Job drawing, mm, ordinate dimensions from the low corner. One solid piece. A direction names the side the tool comes from. Give positions to 0.01 mm unless a question says otherwise; leave off trailing zeros. Order: outer loops, then holes, each group sorted by start corner. A loop starts at its lowest first (then second) coordinate and runs counter-clockwise, first axis right, second up. Notation, with made-up numbers: (-2, -30) - (16, -30) arc R13 cw to (16, -12) - close; hole circle Ø8 at (-4.75, 57.25). An arc over 180 degrees is marked (long way). Use one line per item in the form item = value. Start each with the question number.
1. Band-saw the part on C-C, the plane z = 14.75. List the corners of the cut face in (x, y).
2. Band-saw the part on B-B, the plane x = 23. List the corners of the cut face in (y, z), plus the area to 3 significant figures.
3. Band-saw the part on A-A, the plane y = 23. List the corners of the cut face in (x, z), plus the area to 3 significant figures.
4. Pin check, flat tips, straight feed: P1, Ø1, axis at x = 7, z = 3, coming from the +Y side; P2, Ø2, axis at x = 23.5, z = 17, coming from the +Y side; P3, Ø6, axis at y = 22, z = 3.5, coming from the -X side. Stop position of each tip, or through.
5. Band-saw the part on D-D, the plane z = 6. List the corners of the cut face in (x, y).
6. Pull direction Y, two halves, no side cores. Call the marked faces 4, 5, 6 and 7: +Y half, -Y half, draft (parallel to the pull), parting line (faces both ways), or undercut.
7. Tool access for the marked faces 1, 2 and 3: list every direction of +Z, -Z, +X, -X, +Y, -Y with a clear straight run to the whole face (end or side of a thin tool).
8. Drill centre lines: line 1 (X direction, y = 27, z = 6.25); line 2 (Y direction, x = 23, z = 18.5); line 3 (Y direction, x = 23, z = 12.65). Where is each one in solid material? Low to high.
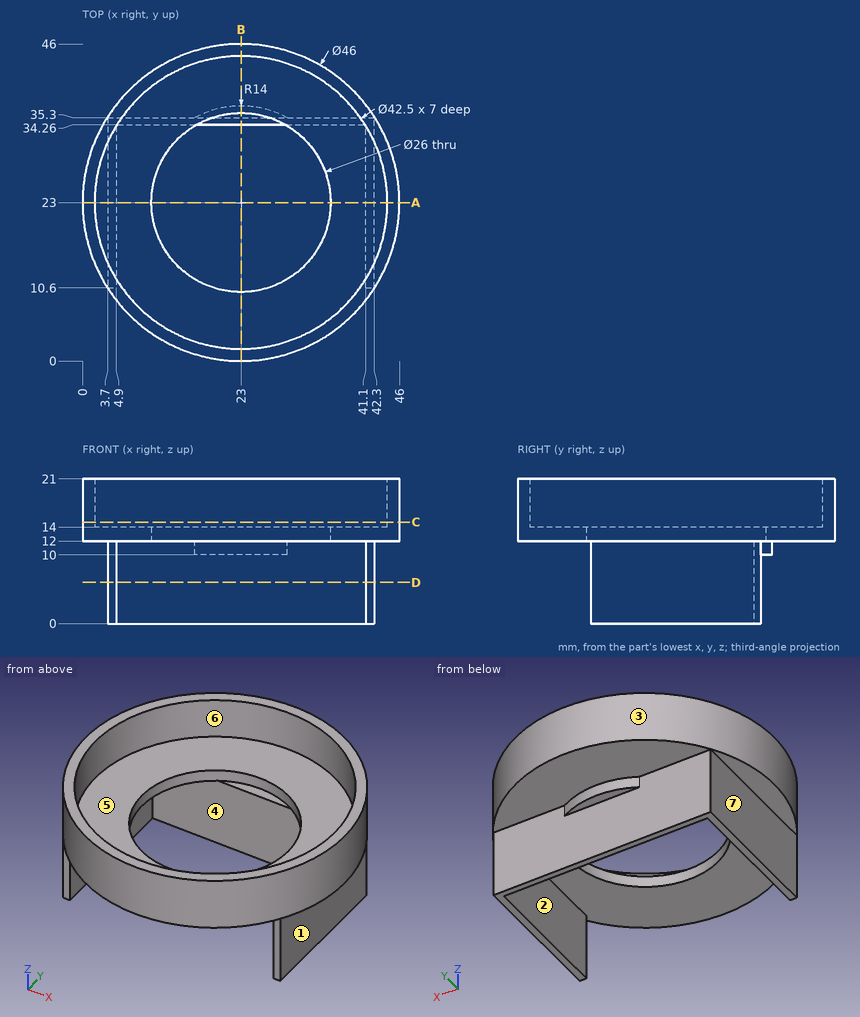
From the geometry:
q1.outline = circle Ø46 at (23, 23); hole circle Ø42.5 at (23, 23)
q2.outline = (0, 12) - (10, 12) - (10, 14) - (1.75, 14) - (1.75, 21) - (0, 21) - close; (34.26, 0) - (35.3, 0) - (35.3, 10) - (37, 10) - (37, 12) - (46, 12) - (46, 21) - (44.25, 21) - (44.25, 14) - (36, 14) - (36, 12) - (34.26, 12) - close
q2.area = 80.4 mm²
q3.outline = (0, 12) - (3.7, 12) - (3.7, 0) - (4.9, 0) - (4.9, 12) - (10, 12) - (10, 14) - (1.75, 14) - (1.75, 21) - (0, 21) - close; (36, 12) - (41.1, 12) - (41.1, 0) - (42.3, 0) - (42.3, 12) - (46, 12) - (46, 21) - (44.25, 21) - (44.25, 14) - (36, 14) - close
q3.area = 93.3 mm²
q4.P1 = 35.3
q4.P2 = 46
q4.P3 = 3.7
q5.outline = (3.7, 10.6) - (4.9, 10.6) - (4.9, 34.26) - (41.1, 34.26) - (41.1, 10.6) - (42.3, 10.6) - (42.3, 35.3) - (3.7, 35.3) - close
q6.face_4 = -Y half
q6.face_5 = undercut
q6.face_6 = undercut
q6.face_7 = draft
q7.face_1 = -Z, +X, +Y, -Y
q7.face_2 = -Z, -Y
q7.face_3 = +Z, -Z
q8.line_1 = 3.7 to 4.9, 41.1 to 42.3
q8.line_2 = 0 to 1.75, 44.25 to 46
q8.line_3 = 0 to 10, 36 to 46
